```python
from build123d import *

# Parameters (mm, degrees)
F0_R     = 6
F1_DEPTH = 25
F3_DEPTH = 20
F4_R     = 30
F5_R     = 15
F6_W     = 8.0703347921
F6_H     = 2.9308869271
F7_DEPTH = 2


with BuildPart() as f1:
    # F0 (on Front) → F1 (new body)
    with BuildSketch(Plane.XZ):
        with BuildLine():
            ThreePointArc((-72.5, 0), (-73.2460947032, 4.2539052968), (-75.3953136439, 8))
            ThreePointArc((-75.3953136439, 8), (-97.5, 0), (-75.3953136439, -8))
            ThreePointArc((-75.3953136439, -8), (-73.2460947032, -4.2539052968), (-72.5, 0))
        make_face()
        with Locations((-85, 0)):
            Circle(F0_R, mode=Mode.SUBTRACT)
        with BuildLine():
            ThreePointArc((-6, -8), (-10, 0), (-6, 8))
            Line((-6, 8), (-75.3953136439, 8))
            ThreePointArc((-75.3953136439, 8), (-73.2460947032, 4.2539052968), (-72.5, 0))
            ThreePointArc((-72.5, 0), (-73.2460947032, -4.2539052968), (-75.3953136439, -8))
            Line((-75.3953136439, -8), (-6, -8))
        make_face()
        with BuildLine():
            ThreePointArc((-6, -8), (4.472135955, -8.94427191), (10, 0))
            ThreePointArc((10, 0), (4.472135955, 8.94427191), (-6, 8))
            ThreePointArc((-6, 8), (-10, 0), (-6, -8))
        make_face()
        Circle(F0_R, mode=Mode.SUBTRACT)
    extrude(amount=F1_DEPTH)

    # F2 (on Top) → F3 (intersect, symmetric)
    with BuildSketch(Plane.XY):
        Polygon((-71.0415363766, -9), (-110.2200075984, -9), (-110.2200075984, -17), (-70.3416270684, -17), (-19.3000906918, -8), (29.2156469077, -8), (29.2156469077, 0), (-20, 0), align=None)
    extrude(amount=F3_DEPTH, both=True, mode=Mode.INTERSECT)

    # F4
    f4_edges = [f1.edges().sort_by_distance(p)[0] for p in [
        (-70.341627, -17, 0),
        (-19.300091, -8, 0),
        (-20, 0, 0),
        (-71.041536, -9, 0),
    ]]
    fillet(f4_edges, radius=F4_R)

    # F5 (call 1 of 4: OpenCascade refuses the feature's edges together)
    f5_edges = [f1.edges().sort_by_distance(p)[0] for p in [
        (-75.395314, -13, 8),
    ]]
    fillet(f5_edges, radius=F5_R)

    # F5#2 (call 2 of 4)
    f5_2_edges = [f1.edges().sort_by_distance(p)[0] for p in [
        (-6, -4, 8),
    ]]
    fillet(f5_2_edges, radius=F5_R)

    # F5#3 (call 3 of 4)
    f5_3_edges = [f1.edges().sort_by_distance(p)[0] for p in [
        (-75.395314, -13, -8),
    ]]
    fillet(f5_3_edges, radius=F5_R)

    # F5#4 (call 4 of 4)
    f5_4_edges = [f1.edges().sort_by_distance(p)[0] for p in [
        (-6, -4, -8),
    ]]
    fillet(f5_4_edges, radius=F5_R)

    # F6 (on face) → F7 (cut)
    with BuildSketch(Plane(origin=(0.7861116292, -4.4582605908, 0), x_dir=(0.984807753, 0.1736481777, 0), z_dir=(0.1736481777, -0.984807753, 0))):
        with Locations((-52.2005781531, 0.226563483)):
            Rectangle(F6_W, F6_H)
    extrude(amount=-F7_DEPTH, mode=Mode.SUBTRACT)


solid = f1.part
```
CAD build for the part. Positions are in the model's coordinates, mm. A direction names the side the tool comes from. Round coordinates to 2 decimals unless told otherwise and drop trailing zeros. Write each loop counter-clockwise with the first axis right and the second up, starting at its lowest first coordinate (ties: lowest second). Pieces come first, ordered by that corner, then holes.
Item 1: Band-saw the part on A-A on x = -85. Write the cut outline in (y, z).
Filled in:
outline: (-17, -12.5) - (-9, -12.5) - (-9, -6) - (-17, -6) - close; (-17, 6) - (-9, 6) - (-9, 12.5) - (-17, 12.5) - close
Item 2: Drop flat-ended pins along their axis: pin 1 Ø2.5 at (x, y) = (-52.5, -12.5) entering from +Z; pin 2 Ø2 at (x, z) = (-69.5, 0.5) entering from +Y; pin 3 Ø2 at (x, z) = (-8, 8.5) entering from -Y; pin 4 Ø11 at (x, z) = (-85, 0) entering from -Y. Give the stop position or say it passes through.
Filled in:
pin 1: stops at z = 8
pin 2: stops at y = -8.55
pin 3: stops at y = -8
pin 4: passes through
Item 3: Band-saw the part on C-C on y = -6.5. Write the cut outline in (x, z), then the cut area to 3 significant figures.
Filled in:
outline: (-56.86, -8) - (-9.8, -8) arc R15 cw to (-3.92, -9.2) arc R10 ccw (long way) to (-3.92, 9.2) arc R15 cw to (-9.8, 8) - (-56.86, 8) - close; hole circle Ø12 at (0, 0)
area: 972 mm2
Item 4: Band-saw the part on D-D on x = 0. Write the cut outline in (y, z).
Filled in:
outline: (-8, -10) - (0, -10) - (0, -6) - (-8, -6) - close; (-8, 6) - (0, 6) - (0, 10) - (-8, 10) - close
Item 5: Drill centre lines: L1, parallel to Z at x = -85, y = -11.5; L2, parallel to Z at x = 0, y = -3; L3, parallel to Y at x = -8, z = 3.75. Where is each one in solid material? Low to high.
Filled in:
L1: z = -12.5 to -6, 6 to 12.5
L2: z = -10 to -6, 6 to 10
L3: y = -8 to 0
Item 6: Mould opens along X. For faces 4 (the cylindrical face through (-70.39, -16.89, 0.12)), 5 (the flat face through (-46.82, -11.85, 0.21)), 6 (the flat face through (-54.767, -13.252, 0.206)), 7 (the flat face through (-45.2, -4.443, 0.112)) say: released by +X, released by -X, zero draft, split by the parting line, or undercut.
Filled in:
face 4: released by +X
face 5: undercut
face 6: undercut
face 7: released by -X
Item 7: Tool access for faces 1 (the flat face through (-39, -8, 8)), 2 (the flat face through (-6.5, -8, 0.1)), 3 (the flat face through (-40, -8, -8)): list every direction of +Z, -Z, +X, -X, +Y, -Y with a clear straight run to the whole face (end or side of a thin tool).
Filled in:
face 1: +Z, +Y, -Y
face 2: +Z, -Z, +X, -Y
face 3: -Z, +Y, -Y
Item 8: Band-saw the part on B-B on z = 0. Write the cut outline in (x, y), then the cut area to 3 significant figures.
Filled in:
outline: (-97.5, -17) - (-91, -17) - (-91, -9) - (-97.5, -9) - close; (-79, -17) - (-72.97, -17) arc R30 ccw to (-67.76, -16.54) - (-54.6, -14.22) - (-54.94, -12.25) - (-46.99, -10.85) - (-46.65, -12.82) - (-21.88, -8.46) arc R30 cw to (-16.68, -8) - (-6, -8) - (-6, 0) - (-17.38, 0) arc R30 ccw to (-22.58, -0.46) - (-68.46, -8.54) arc R30 cw to (-73.67, -9) - (-79, -9) - close; (6, -8) - (10, -8) - (10, 0) - (6, 0) - close
area: 658 mm2
